Answer from the drawing. Dimensions are ordinates in mm from the lowest x, y and z of the part. A direction names the side the tool comes from. Coordinates: 2 decimals unless noted, no trailing zeros. Order: outer loops, then holes, each group sorted by start corner. A loop starts at its lowest first (then second) coordinate and runs counter-clockwise, first axis right, second up. Notation, with made-up numbers: (71, -5.75) -> (102, -5.75) arc R27 cw to (102, 26.25) -> close; hole circle Ø9 at (56.25, 2). An arc over 180 degrees is marked (long way). Use CSV: the item, a comma, the result in double quotes.
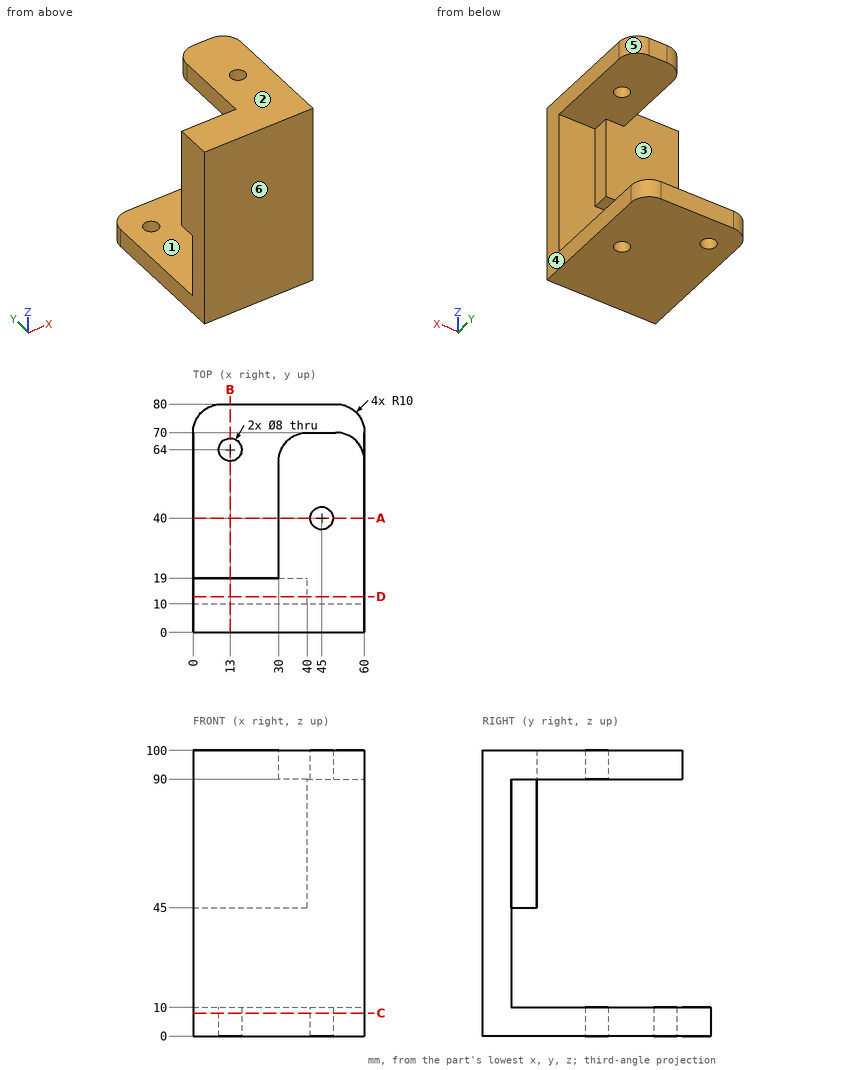
Item 1: The mould has two halves that part along Z. Classify the marked faces 1, 2, 3 and 4: +Z half, -Z half, draft (parallel to the pull), parting line (faces both ways), or undercut.
Return value:
face 1,"undercut"
face 2,"+Z half"
face 3,"undercut"
face 4,"draft"
Item 2: Straight lines are drawn through the part: line 1 along Z through (x, y) = (38, 29.5); line 2 along Y through (x, z) = (45, 7.25); line 3 along Z through (x, y) = (8.5, 44). For each, find the intervals that lie inside material, in ascending order.
Return value:
line 1,"z = 0 to 10, 90 to 100"
line 2,"y = 0 to 36, 44 to 80"
line 3,"z = 0 to 10"
Item 3: Find section B-B, the plane x = 13. Give the vertices of the cut face in (y, z), then the cut area to 4 significant figures.
Return value:
outline,"(0, 0) -> (60, 0) -> (60, 10) -> (10, 10) -> (10, 45) -> (19, 45) -> (19, 100) -> (0, 100) -> close; (68, 0) -> (80, 0) -> (80, 10) -> (68, 10) -> close"
area,"2,115 mm^2"
Item 4: Find section C-C, the plane z = 8. Give the vertices of the cut face in (x, y).
Return value:
outline,"(0, 0) -> (60, 0) -> (60, 70) arc R10 ccw to (50, 80) -> (10, 80) arc R10 ccw to (0, 70) -> close; hole circle Ø8 at (13, 64); hole circle Ø8 at (45, 40)"
Item 5: Find section D-D, the plane y = 12.5. Give the vertices of the cut face in (x, z).
Return value:
outline,"(0, 0) -> (60, 0) -> (60, 10) -> (0, 10) -> close; (0, 45) -> (40, 45) -> (40, 90) -> (60, 90) -> (60, 100) -> (0, 100) -> close"
Item 6: Find section A-A, the plane y = 40. Give the vertices of the cut face in (x, z), then the cut area to 3 significant figures.
Return value:
outline,"(0, 0) -> (41, 0) -> (41, 10) -> (0, 10) -> close; (30, 90) -> (41, 90) -> (41, 100) -> (30, 100) -> close; (49, 0) -> (60, 0) -> (60, 10) -> (49, 10) -> close; (49, 90) -> (60, 90) -> (60, 100) -> (49, 100) -> close"
area,"740 mm^2"
Item 7: Each of these flat-tipped pins is pushed along its axis until it touches: P1, Ø3, axis at x = 47.5, z = 95, coming from the +Y side; P2, Ø5, axis at x = 24, y = 57, coming from the +Z side; P3, Ø8, axis at x = 24, z = 73, coming from the -Y side; P4, Ø6.5, axis at x = 45, y = 40, coming from the +Z side. Where does it stop, or does it pass through?
Return value:
P1,"stops at y = 70"
P2,"stops at z = 10"
P3,"stops at y = 0"
P4,"passes through"
Item 8: A tool of negligible diameter and unlimited length cuts with its end or side. For the marked faces 5 and 6, from which of +Z, -Z, +X, -X, +Y, -Y can it reach the whole face along a straight path? Write none if from no direction.
Return value:
face 5,"+Z, +X, +Y"
face 6,"+Z, -Z, +X, -X, -Y"
